The model under review builds one solid part; all positions refer to its coordinate system, in mm. A direction names the side the tool comes from. Give positions to 0.01 mm unless a question says otherwise; leave off trailing zeros. Order: outer loops, then holes, each group sorted by start corner. A loop starts at its lowest first (then second) coordinate and runs counter-clockwise, first axis right, second up.
Autodesk Inventor part; units mm, degrees
ref_plane "YZ Plane" through (0, 0, 0) normal (1, 0, 0) x (0, 1, 0)
ref_plane "XZ Plane" through (0, 0, 0) normal (0, 1, 0) x (-1, 0, 0)
ref_plane "XY Plane" through (0, 0, 0) normal (0, 0, 1) x (1, 0, 0)
sketch "Sketch1" plane through (0, 0, 0) normal (1, 0, 0) x (0, 1, 0)
  line L0 (33.4134, 34.8656) -> (-36.4366, 34.8656)
  line L1 (-36.4366, 34.8656) -> (-36.4366, -22.2844)
  line L2 (-36.4366, -22.2844) -> (33.4134, -22.2844)
  line L3 (33.4134, -22.2844) -> (33.4134, 34.8656)
  point P0 (0, 0)
  dimension "d0" = 57.15
  dimension "d1" = 69.85
extrude "Extrusion1" add sketch "Sketch1" along normal blind 12.7
sketch "Sketch2" plane through (12.7, 0, 0) normal (1, 0, 0) x (0, 0, -1)
  line L0 (-34.8656, 8.0134) -> (22.2844, 8.0134)
  line L1 (22.2844, 8.0134) -> (22.2844, -11.0366)
  line L2 (22.2844, -11.0366) -> (-34.8656, -11.0366)
  line L3 (-34.8656, -11.0366) -> (-34.8656, 8.0134)
  line L4 (22.2844, -36.4366) -> (22.2844, 33.4134)
  line L5 (-34.8656, 33.4134) -> (-34.8656, -36.4366)
  line L6 (22.2844, 33.4134) -> (-34.8656, 33.4134)
  point P0 (0, 0)
  dimension "d5" = 0
  dimension "d9" = 57.15
  dimension "d16" = 19.05
  dimension "d17" = 25.4
extrude "Extrusion2" add sketch "Sketch2" along normal blind 57.15 contours L0 L1 L2 L3
fillet "Fillet1" radius 28.575 1 edges at (69.85, -1.5116, 34.8656)
fillet "Fillet2" radius 28.575 1 edges at (69.85, -1.5116, -22.2844)
sketch "Sketch3" plane through (12.7, 8.0134, 34.8656) normal (0, 1, 0) x (1, 0, 0)
  circle A0 centre (28.575, 28.575) radius 19.812
  line L0 (0, 0) -> (28.575, 0)
  line L1 (0, 57.15) -> (0, 0)
  point P0 (-12.7, 34.8656)
  dimension "d11" = 39.624
  dimension "d12" = 28.575
  dimension "d13" = 28.575
extrude "Extrusion3" cut sketch "Sketch3" against normal blind 50.8
sketch "Sketch4" plane through (12.7, 0, 0) normal (1, 0, 0) x (0, 0, -1)
  point P0 (0, 0)
sketch "Sketch5" plane through (12.7, 0, 0) normal (1, 0, 0) x (0, 0, -1)
  line L0 (22.2844, -36.4366) -> (22.2844, 33.4134)
  line L1 (22.2844, 33.4134) -> (-34.8656, 33.4134)
  point P0 (0, 0)
  point P1 (-6.2906, 20.7134)
  dimension "d25" = 28.575
  dimension "d35" = 12.7
hole "Hole1" at (12.7, 20.7134, 6.2906) direction (-1, 0, 0) diameter 8.4328 end through all counterbore diameter 15.875 counterbore depth 4.7625
sketch "Sketch6" plane through (12.7, 0, 0) normal (1, 0, 0) x (0, 0, -1)
  line L0 (22.2844, -36.4366) -> (22.2844, 33.4134)
  line L1 (-34.8656, -36.4366) -> (22.2844, -36.4366)
  point P0 (0, 0)
  point P1 (-6.2906, -23.7366)
  dimension "d33" = 28.575
  dimension "d34" = 12.7
hole "Hole2" at (12.7, -23.7366, 6.2906) direction (-1, 0, 0) diameter 8.4328 end through all counterbore diameter 15.875 counterbore depth 4.7625
properties part number "Organic Filter Holder"
Item 1: Take a section at C-C (y = 17.5). Give the boundary of the cut face in (x, z), and give its area (3 significant figures).
Values found:
outline: (0, -22.28) - (12.7, -22.28) - (12.7, -0.97) - (7.94, -0.97) - (7.94, 3.56) - (0, 3.56) - close; (0, 9.02) - (7.94, 9.02) - (7.94, 13.55) - (12.7, 13.55) - (12.7, 34.87) - (0, 34.87) - close
area: 613 mm2
Item 2: For line 1 (Y direction, x = 8, z = 11.5); line 2 (Y direction, x = 17, z = 11.5); line 3 (X direction, y = 29.5, z = -5.5), list the stretches that pass through material, from the lowest coordinate up.
Values found:
line 1: y = -36.44 to -29.73, -17.75 to 14.72, 26.7 to 33.41
line 2: y = -11.04 to 8.01
line 3: x = 0 to 12.7
Item 3: For faces 5 (the cylindrical face through (10.29, 15.35, 12.14)), 6 (the flat face through (22, -11.037, 12)), 7 (the flat face through (22, 8.013, 13)), list the 3-axis set-ups (+Z, -Z, +X, -X, +Y, -Y) from which the entire face can be reached by the end or side of a thin tool; tool diameter is ignored.
Values found:
face 5: +X
face 6: +Z, -Z, +X, -Y
face 7: +Z, -Z, +X, +Y
Item 4: Take a section at B-B (x = 44). Give the boundary of the cut face in (y, z).
Values found:
outline: (-11.04, -22.15) - (8.01, -22.15) - (8.01, -13.33) - (-11.04, -13.33) - close; (-11.04, 25.91) - (8.01, 25.91) - (8.01, 34.74) - (-11.04, 34.74) - close
Item 5: Take a section at D-D (x = 34.5). Give the boundary of the cut face in (y, z).
Values found:
outline: (-11.04, -22.28) - (8.01, -22.28) - (8.01, -12.33) - (-11.04, -12.33) - close; (-11.04, 24.91) - (8.01, 24.91) - (8.01, 34.87) - (-11.04, 34.87) - close
Item 6: Take a section at A-A (z = 12). Give the boundary of the cut face in (x, y), and give its area (3 significant figures).
Values found:
outline: (0, -36.44) - (12.7, -36.44) - (12.7, -29.25) - (7.94, -29.25) - (7.94, -18.22) - (12.7, -18.22) - (12.7, -11.04) - (22.3, -11.04) - (22.3, 8.01) - (12.7, 8.01) - (12.7, 15.2) - (7.94, 15.2) - (7.94, 26.23) - (12.7, 26.23) - (12.7, 33.41) - (0, 33.41) - close; (60.25, -11.04) - (69.27, -11.04) - (69.27, 8.01) - (60.25, 8.01) - close
area: 1,140 mm2
Item 7: Draft analysis for pull direction Z (two halves, no side actions). For faces 1 (the flat face through (7.938, 24, 3)), 2 (the cylindrical face through (61.257, -1.645, -14.136)), 3 (the flat face through (12.7, 12, 7)), 4 (the flat face through (7.938, -20, 3)), state which applies: released by +Z, released by -Z, zero draft, split by the parting line, or undercut.
Values found:
face 1: undercut
face 2: released by -Z
face 3: zero draft
face 4: undercut
Item 8: Clearance check with flat-ended pins moving along their axes: pin 1 Ø7.5 at (y, z) = (-22, 0.5) entering from +X; pin 2 Ø5 at (x, z) = (59.5, 26.5) entering from -Y; pin 3 Ø10 at (x, z) = (57, 6) entering from +Y. State where each tip first meets the part, or that it passes through.
Values found:
pin 1: stops at x = 12.7
pin 2: stops at y = -11.04
pin 3: stops at y = 8.01
